from build123d import *

# Parameters (mm, degrees)
SKETCH1_R           = 40
BOSS_EXTRUDE1_DEPTH = 1.6
SKETCH2_R           = 7.5
SKETCH2_R_2         = 2
CUT_EXTRUDE1_DEPTH  = 1.6
CHAMFER1_SIZE       = 1.6


with BuildPart() as part:
    # Sketch1 → Boss-Extrude1 (new body)
    with BuildSketch(Plane.XY):
        Circle(SKETCH1_R)
    extrude(amount=BOSS_EXTRUDE1_DEPTH)

    # Sketch2 → Cut-Extrude1 (cut)
    with BuildSketch(Plane.XY.offset(1.6)):
        Circle(SKETCH2_R)
        with Locations((0, 22)):
            Circle(SKETCH2_R_2)
        with Locations((19.052558883, -11)):
            Circle(SKETCH2_R_2)
        with Locations((-19.052558883, -11)):
            Circle(SKETCH2_R_2)
    extrude(amount=-CUT_EXTRUDE1_DEPTH, mode=Mode.SUBTRACT)

    # Chamfer1
    chamfer1_edges = [part.edges().sort_by_distance(p)[0] for p in [
        (-40, 0, 1.6),
    ]]
    chamfer(chamfer1_edges, length=CHAMFER1_SIZE - 0.0001)  # a hair under: the kernel refuses the full size


solid = part.part
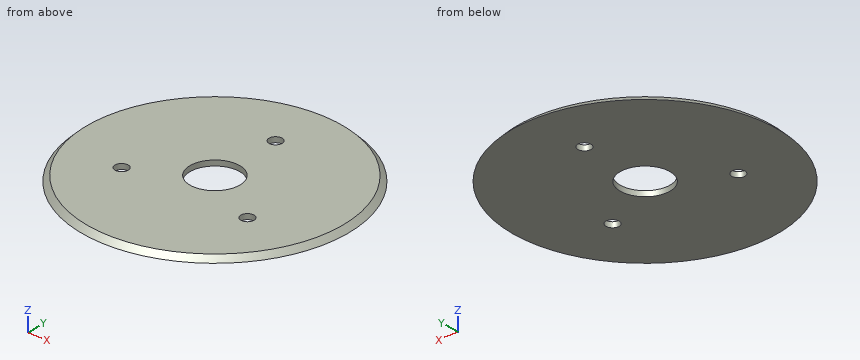
Could you check a few things on this model? Use its own coordinates, in mm. Give positions to 0.01 mm unless a question says otherwise; leave off trailing zeros. Write each loop counter-clockwise with the first axis right and the second up, starting at its lowest first coordinate (ties: lowest second). Pieces come first, ordered by that corner, then holes. Notation, with made-up numbers: (50, 16.5) -> (105, 16.5) arc R7 ccw to (105, 20.5) -> close; hole circle Ø9 at (46, 15.25). An arc over 180 degrees is marked (long way). Answer as a JSON object with one key per item and string values.
Q1. Suppose I cut it at A-A on x = 0. Count the separate pieces of the cut face and the enclosed holes in it, then the cut area to 3 significant figures.
Taken from the geometry:
{"separate pieces": "3", "enclosed holes": "0", "area": "95.0 mm²"}
Q2. Suppose I cut it at C-C on z = 0.55. Write out the boundary of the cut face in (x, y), then the cut area to 3 significant figures.
Taken from the geometry:
{"outline": "circle Ø78.9 at (0, 0); hole circle Ø4 at (-19.05, -11); hole circle Ø15 at (0, 0); hole circle Ø4 at (0, 22); hole circle Ø4 at (19.05, -11)", "area": "4,670 mm²"}
Q3. Please list where these lines run through material, in increasing order: L1, parallel to Y at x = 0, z = 0.75; L2, parallel to X at y = -12, z = 0.85; L3, parallel to Y at x = 0.5, z = 0.8.
Taken from the geometry:
{"L1": "y = -39.25 to -7.5, 7.5 to 20, 24 to 39.25", "L2": "x = -37.27 to -20.78, -17.32 to 17.32, 20.78 to 37.27", "L3": "y = -39.2 to -7.48, 7.48 to 20.06, 23.94 to 39.2"}
